The model under review builds one solid part; all positions refer to its coordinate system, in mm. A direction names the side the tool comes from. Give positions to 0.01 mm unless a question says otherwise; leave off trailing zeros. Order: outer loops, then holes, each group sorted by start corner. A loop starts at its lowest first (then second) coordinate and runs counter-clockwise, first axis right, second up.
```python
from build123d import *

# Parameters (mm, degrees)
F1_DEPTH = 18
F2_DEPTH = 15
F3_DEPTH = 15
F4_DEPTH = 15


# Not quite as in the source:
# - the program builds the solid bodies; features that only make, move or delete a surface that nothing else refers to are left out


with BuildPart() as f1:
    # F0 (on Top) → F1 (new body, symmetric)
    with BuildSketch(Plane.XY):
        Polygon((22.5, 12.9903810568), (-22.5, 12.9903810568), (0, -25.9807621135), align=None)
    extrude(amount=F1_DEPTH, both=True)

    # F2 (add): a face of the model
    f2_faces = [f1.faces().sort_by_distance(p)[0] for p in [
        (11.25, -6.4951905284, 0),
    ]]
    extrude(f2_faces, amount=F2_DEPTH)

    # F3 (add): a face of the model
    f3_faces = [f1.faces().sort_by_distance(p)[0] for p in [
        (0, 12.9903810568, 0),
    ]]
    extrude(f3_faces, amount=F3_DEPTH)

    # F4 (add): a face of the model
    f4_faces = [f1.faces().sort_by_distance(p)[0] for p in [
        (-11.25, -6.4951905284, 0),
    ]]
    extrude(f4_faces, amount=F4_DEPTH)


solid = f1.part
```
Item 1: For line 1 (Y direction, x = 0, z = -8); line 2 (X direction, y = 15.5, z = 8.5); line 3 (X direction, y = -29.5, z = 7), list the stretches that pass through material, from the lowest coordinate up.
Values found:
line 1: y = -25.98 to 27.99
line 2: x = -22.5 to 22.5
line 3: x = -15.29 to -6.1, 6.1 to 15.29
Item 2: Take a section at A-A (z = 2.5). Give the boundary of the cut face in (x, y), and give its area (3 significant figures).
Values found:
outline: (-35.49, 5.49) - (-12.99, -33.48) - (0, -25.98) - (12.99, -33.48) - (35.49, 5.49) - (22.5, 12.99) - (22.5, 27.99) - (-22.5, 27.99) - (-22.5, 12.99) - close
area: 2,900 mm2
Item 3: Take a section at B-B (y = 14.5). Give the boundary of the cut face in (x, z).
Values found:
outline: (-22.5, -18) - (22.5, -18) - (22.5, 18) - (-22.5, 18) - close
Item 4: Take a section at C-C (x = -10.5). Give the boundary of the cut face in (y, z), and give its area (3 significant figures).
Values found:
outline: (-32.04, -18) - (27.99, -18) - (27.99, 18) - (-32.04, 18) - close
area: 2,160 mm2
Item 5: Clearance check with flat-ended pins moving along their axes: pin 1 Ø12 at (x, z) = (6.5, 9.5) entering from -Y; pin 2 Ø2 at (y, z) = (-24.5, -11) entering from -X; pin 3 Ø4 at (y, z) = (1.5, -2.5) entering from +X. State where each tip first meets the part, or that it passes through.
Values found:
pin 1: stops at y = -33.2
pin 2: stops at x = -18.75
pin 3: stops at x = 34.34
Item 6: For faces 1 (the flat face through (-6.404, -29.678, 0.252)), 2 (the flat face through (22.5, 20, 0)), 3 (the flat face through (-22.5, 20, 0)), list the 3-axis set-ups (+Z, -Z, +X, -X, +Y, -Y) from which the entire face can be reached by the end or side of a thin tool; tool diameter is ignored.
Values found:
face 1: +Z, -Z, -Y
face 2: +Z, -Z, +X, +Y
face 3: +Z, -Z, -X, +Y
Item 7: Draft analysis for pull direction X (two halves, no side actions). For faces 4 (the flat face through (0, 27.99, 0)), 5 (the flat face through (28.904, 9.293, 0.252)), 6 (the flat face through (6.404, -29.678, 0.252)), state which applies: released by +X, released by -X, zero draft, split by the parting line, or undercut.
Values found:
face 4: zero draft
face 5: released by +X
face 6: undercut
